The model under review builds one solid part; all positions refer to its coordinate system, in mm. Face numbers are marked on the shaded views. A direction names the side the tool comes from. Give positions to 0.01 mm unless a question says otherwise; leave off trailing zeros. Loops run counter-clockwise (first coordinate to the right, second up) from the corner with the lowest first, then second, coordinate; pieces in that order, holes last. Notation, with made-up numbers: M 72.5,26.5 L 104.5,26.5 A25 ccw 104.5,62.5 Z; hole C -23.75,51.25 d7. An arc over 180 degrees is marked long. Return JSON: item names as keys, results as strings.
Autodesk Fusion 360 part; units mm, degrees
sketch "Skizze1" plane through (0, 0, 0) normal (0, 0, 1) x (1, 0, 0)
  line L0 (11.5, 5.75) -> (-11.5, 5.75)
  line L1 (-11.5, 5.75) -> (-11.5, -5.75)
  line L2 (-11.5, -5.75) -> (11.5, -5.75)
  line L3 (11.5, -5.75) -> (11.5, 5.75)
  line L4 (11.5, 5.75) -> (-11.5, -5.75) construction
  line L5 (-11.5, 5.75) -> (11.5, -5.75) construction
  dimension "d1" = 11.5
  dimension "d2" = 23
extrude "Extrusion1" add sketch "Skizze1" along normal mid plane 20
sketch "Skizze2" plane through (0, 5.75, 0) normal (0, 1, 0) x (-1, 0, 0)
  line L0 (11.5, -10) -> (11.5, 10)
  line L1 (11.5, 10) -> (-11.5, 10)
  line L2 (-11.5, 10) -> (-11.5, -10)
  line L3 (-11.5, -10) -> (11.5, -10)
  line L4 (16.5, -7.5) -> (-16.5, -7.5)
  line L5 (-16.5, -7.5) -> (-16.5, -6.5)
  line L6 (-16.5, -6.5) -> (16.5, -6.5)
  line L7 (16.5, -6.5) -> (16.5, -7.5)
  dimension "d5" = 2.5
  dimension "d6" = 1
  dimension "d7" = 5
  dimension "d8" = 5
extrude "Extrusion2" add sketch "Skizze2" against normal blind 11.5 contours L0 L4 L6 L7 | L2 L4 L5 L6
sketch "Skizze3" plane through (0, 0, -10) normal (0, 0, -1) x (-1, 0, 0)
  line L0 (-11.5, 5.75) -> (-11.5, -5.75)
  line L1 (-11.5, -5.75) -> (11.5, -5.75)
  line L2 (11.5, -5.75) -> (11.5, 5.75)
  line L3 (11.5, 5.75) -> (-11.5, 5.75)
  circle A0 centre (5.75, 0) radius 5.75
  circle A1 centre (-0.5, 0) radius 3
  dimension "d11" = 11.5
  dimension "d13" = 6
  dimension "d14" = 12
extrude "Extrusion3" add sketch "Skizze3" along normal blind 4 contours A0 A1 | A0 A1 | A0 A1
fillet "Abrundung1" radius 1 2 edges at (-0.7, 2.7495, -12) (-0.7, -2.7495, -12)
sketch "Skizze4" plane through (0, 0, -14) normal (0, 0, -1) x (-1, 0, 0)
  arc A0 (1.0733, -3.3453) -> (1.0733, 3.3453) centre (5.75, 0) ccw
  arc A1 (0.07, 2.9454) -> (1.0733, 3.3453) centre (0.26, 3.9271) ccw
  arc A2 (0.07, 2.9454) -> (0.07, -2.9454) centre (-0.5, 0) ccw
  arc A3 (1.0733, -3.3453) -> (0.07, -2.9454) centre (0.26, -3.9271) ccw
  circle A4 centre (5.75, 0) radius 2.5
  dimension "d19" = 5
extrude "Extrusion4" add sketch "Skizze4" along normal blind 2 contours A4
sketch "Skizze5" plane through (0, 0, -16) normal (0, 0, -1) x (-1, 0, 0)
  circle A0 centre (5.75, 0) radius 2.5
  line L0 (7.75, 8.5) -> (3.75, 8.5)
  line L1 (3.75, -8.5) -> (7.75, -8.5)
  line L2 (7.75, 8.5) -> (3.75, -8.5) construction
  line L3 (3.75, 8.5) -> (7.75, -8.5) construction
  line L4 (-2.75, 2) -> (-2.75, -2)
  line L5 (14.25, -2) -> (14.25, 2)
  line L6 (14.25, 2) -> (-2.75, -2) construction
  line L7 (-2.75, 2) -> (14.25, -2) construction
  line L8 (3.75, 2) -> (-2.75, 2)
  line L9 (3.75, 8.5) -> (3.75, 2)
  line L10 (3.75, 0.4706) -> (3.75, -0.4706)
  line L11 (3.75, -2) -> (3.75, -8.5)
  line L12 (-2.75, -2) -> (3.75, -2)
  line L13 (7.75, -2) -> (14.25, -2)
  line L14 (7.75, -8.5) -> (7.75, -2)
  line L15 (7.75, -0.4706) -> (7.75, 0.4706)
  line L16 (7.75, 2) -> (7.75, 8.5)
  line L17 (14.25, 2) -> (7.75, 2)
  line L18 (6.2206, 2) -> (5.2794, 2)
  point P0 (5.75, 0)
  point P1 (5.75, 0)
  dimension "d22" = 4
  dimension "d23" = 17
extrude "Extrusion5" add sketch "Skizze5" along normal blind 1 contours A0 | L0 L1 L4 L5 L8 L9 L11 L12 L13 L14 L16 L17
fillet "Abrundung2" radius 2 8 edges at (2.75, -2, -16.5) (-3.75, -8.5, -16.5) (-7.75, -8.5, -16.5) (-14.25, -2, -16.5) (-14.25, 2, -16.5) (-7.75, 8.5, -16.5) (-3.75, 8.5, -16.5) (2.75, 2, -16.5)
sketch "Skizze6" plane through (0, 0, -17) normal (0, 0, -1) x (-1, 0, 0)
  arc A0 (-0.75, 2) -> (-0.75, -2) centre (-0.75, 0) ccw
  line L0 (-0.75, -2) -> (3.75, -2)
  line L1 (3.75, -2) -> (3.75, -6.5)
  arc A1 (3.75, -6.5) -> (7.75, -6.5) centre (5.75, -6.5) ccw
  line L2 (7.75, -6.5) -> (7.75, -2)
  line L3 (7.75, -2) -> (12.25, -2)
  arc A2 (12.25, -2) -> (12.25, 2) centre (12.25, 0) ccw
  line L4 (12.25, 2) -> (7.75, 2)
  line L5 (7.75, 2) -> (7.75, 6.5)
  arc A3 (7.75, 6.5) -> (3.75, 6.5) centre (5.75, 6.5) ccw
  line L6 (3.75, 6.5) -> (3.75, 2)
  line L7 (3.75, 2) -> (-0.75, 2)
  line L8 (5.75, 6.5) -> (5.75, -6.5) construction
  line L9 (12.25, 0) -> (-0.75, 0) construction
  circle A4 centre (5.75, 0) radius 2
  dimension "d28" = 4
extrude "Extrusion6" add sketch "Skizze6" along normal blind 1 contours A4
sketch "Skizze7" plane through (-11.5, 0, 0) normal (-1, 0, 0) x (0, 0, 1)
  line L0 (-6.5, 5.75) -> (-6.5, -5.75)
  line L1 (-6.5, -5.75) -> (10, -5.75)
  line L2 (10, -5.75) -> (10, 5.75)
  line L3 (10, 5.75) -> (-6.5, 5.75)
  ellipse E0 centre (6, 0) end of major axis (6, 2.5) minor radius 1.5
  line L4 (6, -2.5) -> (6, 2.5)
  line L5 (7.5, 0) -> (4.5, 0)
  dimension "d31" = 5
  dimension "d32" = 3
  dimension "d33" = 4
extrude "Extrusion7" add sketch "Skizze7" along normal blind 2 contours E0 L4 L5 | E0 L4 L5 | E0 L4 L5 | E0 L4 L5
equation "d8 = d7"
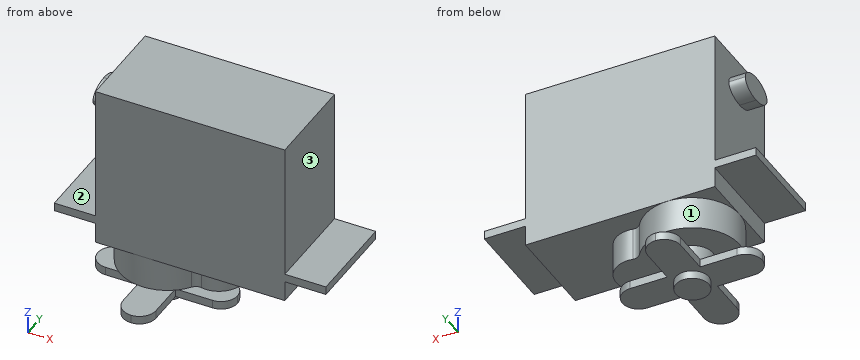
1) Consider section B-B on y = 5.25. Write out the cut boundary in (x, z).
From the geometry:
{"outline": "M -16.5,-7.5 L -11.5,-7.5 L -11.5,-10 L -8.1,-10 L -8.1,-14 L -3.4,-14 L -3.4,-10 L 11.5,-10 L 11.5,-7.5 L 16.5,-7.5 L 16.5,-6.5 L 11.5,-6.5 L 11.5,10 L -11.5,10 L -11.5,-6.5 L -16.5,-6.5 Z; M -7.75,-17 L -3.75,-17 L -3.75,-16 L -7.75,-16 Z"}
2) Tool access review of the marked faces 1, 2 and 3: name each direction out of +Z, -Z, +X, -X, +Y, -Y from which nothing blocks a thin tool from reaching the whole face with its end or side.
From the geometry:
{"face 1": "none", "face 2": "-X, +Y, -Y", "face 3": "+Z, +X, +Y, -Y"}
3) Consider section C-C on z = -15. Write out the cut boundary in (x, y).
From the geometry:
{"outline": "C -5.75,0 d5"}
4) Insertion check: pin 1 (1.5 mm diameter, centred on x = -9, y = 1, fed in from -Z); pin 2 (4 mm diameter, centred on x = 15, y = 1, fed in from +Z); pin 3 (6 mm diameter, centred on x = -7.5, z = 2.5, fed in from -Y). Each pin has a flat end and moves straight along its axis. Give the tip position at first contact, or say it passes through.
From the geometry:
{"pin 1": "z = -17", "pin 2": "z = -6.5", "pin 3": "y = -5.75"}
5) Wall thickness on L1, parallel to Z at x = -5.5, y = 5; L2, parallel to Z at x = -14.5, y = 2; L3, parallel to Y at x = -4.5, z = -0.25: over which ranges is each line inside the solid? List them lowest first. Write a range as from..to.
From the geometry:
{"L1": "-17..-16, -14..10", "L2": "-7.5..-6.5", "L3": "-5.75..5.75"}
6) Consider section A-A on x = -11. Write out the cut boundary in (y, z), then the cut area to 3 significant figures.
From the geometry:
{"outline": "M -5.75,-10 L -2.35,-10 L -2.35,-14 L 2.35,-14 L 2.35,-10 L 5.75,-10 L 5.75,10 L -5.75,10 Z; M -2,-17 L 2,-17 L 2,-16 L -2,-16 Z", "area": "253 mm²"}
7) Consider section D-D on x = -2.5. Write out the cut boundary in (y, z).
From the geometry:
{"outline": "M -5.75,-10 L -4.74,-10 L -4.74,-14 L 4.74,-14 L 4.74,-10 L 5.75,-10 L 5.75,10 L -5.75,10 Z; M -2,-17 L 2,-17 L 2,-16 L -2,-16 Z"}
